The figure shows three views and two pictorial views of one solid part (mm, origin at its lowest corner). Answer the questions. A direction names the side the tool comes from. Give positions to 0.01 mm unless a question says otherwise; leave off trailing zeros. Order: outer loops, then holes, each group sorted by start corner. A loop starts at its lowest first (then second) coordinate and runs counter-clockwise, first axis right, second up. Notation, with made-up numbers: (-33, 13) - (-8, 13) arc R19 cw to (-8, 39) - close; hole circle Ø6 at (77, -19). An arc over 180 degrees is marked (long way). Return JSON: item names as keys, results as strings. Group by question number.
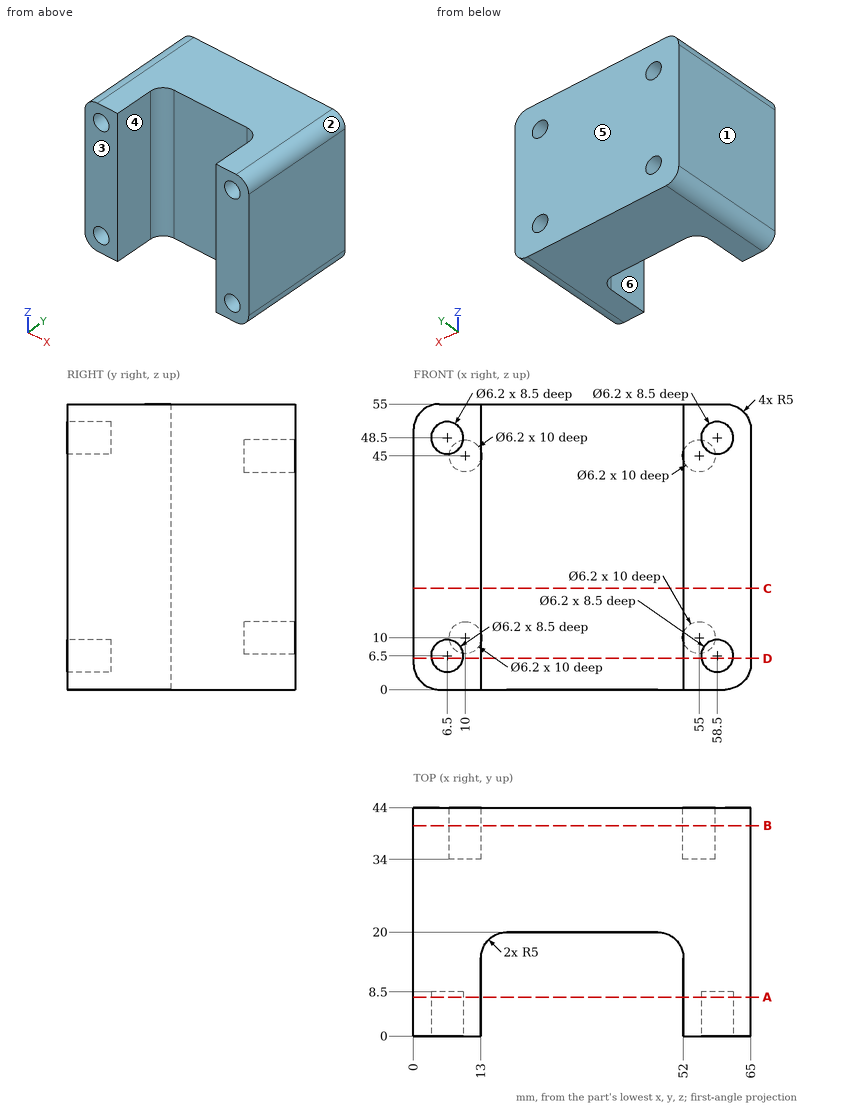
1. The part is cut by section B-B (y = 40.5). Give the vertices of the cut face in (x, z), and give its area (3 significant figures).
2. Determine the mould class of the marked faces 1, 2, 3 and 4 for opening direction X: released by +X, released by -X, zero draft, split by the parting line, or undercut.
3. A tool of negligible diameter and unlimited length cuts with its end or side. For the marked faces 5 and 6, from which of +Z, -Z, +X, -X, +Y, -Y can it reach the whole face along a straight path? Write none if from no direction.
4. Each of these flat-tipped pins is pushed along its axis until it touches: pin 1 (1.9 mm diameter, centred on x = 58.5, z = 47.5, fed in from -Y); pin 2 (1.5 mm diameter, centred on x = 8, z = 9.5, fed in from +Y); pin 3 (1.5 mm diameter, centred on x = 44.5, z = 18.5, fed in from -Y). Where does it stop, or does it pass through?
5. The part is cut by section A-A (y = 7.5). Give the vertices of the cut face in (x, z), and give its area (3 significant figures).
6. The part is cut by section C-C (z = 19.5). Give the vertices of the cut face in (x, y), and give its area (3 significant figures).
7. Consider probe 1 along X at (y, z) = (36.75, 45); probe 2 along X at (y, z) = (11, 43); probe 3 along Z at (x, y) = (58, 4). Determine where each line is inside the solid, lowest interval first. Write a range as from..to.
8. The part is cut by section D-D (z = 6). Give the vertices of the cut face in (x, y).
Answers:
{
 "1": {"outline": "(0, 5) arc R5 ccw to (5, 0) - (60, 0) arc R5 ccw to (65, 5) - (65, 50) arc R5 ccw to (60, 55) - (5, 55) arc R5 ccw to (0, 50) - close; hole circle Ø6.2 at (10, 10); hole circle Ø6.2 at (10, 45); hole circle Ø6.2 at (55, 10); hole circle Ø6.2 at (55, 45)", "area": "3,430 mm^2"},
 "2": {"face 1": "released by -X", "face 2": "released by +X", "face 3": "zero draft", "face 4": "undercut"},
 "3": {"face 5": "+Z, -Z, +X, -X, +Y", "face 6": "+Z, -Z, -Y"},
 "4": {"pin 1": "stops at y = 8.5", "pin 2": "stops at y = 34", "pin 3": "stops at y = 20"},
 "5": {"outline": "(0, 5) arc R5 ccw to (5, 0) - (13, 0) - (13, 55) - (5, 55) arc R5 ccw to (0, 50) - close; (52, 0) - (60, 0) arc R5 ccw to (65, 5) - (65, 50) arc R5 ccw to (60, 55) - (52, 55) - close; hole circle Ø6.2 at (6.5, 6.5); hole circle Ø6.2 at (6.5, 48.5); hole circle Ø6.2 at (58.5, 6.5); hole circle Ø6.2 at (58.5, 48.5)", "area": "1,290 mm^2"},
 "6": {"outline": "(0, 0) - (13, 0) - (13, 15) arc R5 cw to (18, 20) - (47, 20) arc R5 cw to (52, 15) - (52, 0) - (65, 0) - (65, 44) - (0, 44) - close", "area": "2,090 mm^2"},
 "7": {"probe 1": "x = 0..6.9, 13.1..51.9, 58.1..65", "probe 2": "x = 0..13, 52..65", "probe 3": "z = 0..3.44, 9.56..45.44, 51.56..55"},
 "8": {"outline": "(0, 0) - (3.44, 0) - (3.44, 8.5) - (9.56, 8.5) - (9.56, 0) - (13, 0) - (13, 15) arc R5 cw to (18, 20) - (47, 20) arc R5 cw to (52, 15) - (52, 0) - (55.44, 0) - (55.44, 8.5) - (61.56, 8.5) - (61.56, 0) - (65, 0) - (65, 44) - (0, 44) - close"}
}
